Verification items for the finished model (mm, model axes). Face numbers are marked on the shaded views. Give positions to 0.01 mm unless a question says otherwise; leave off trailing zeros. Write each loop counter-clockwise with the first axis right and the second up, starting at its lowest first coordinate (ties: lowest second). Pieces come first, ordered by that corner, then holes. Notation, with made-up numbers: (41, -0.5) -> (53, -0.5) arc R21 cw to (53, 16.5) -> close; hole circle Ø6 at (-13, 8). An arc over 180 degrees is marked (long way). Use one line per item in the form item = value. Start each with the question number.
(1) Depth check by flat-ended pin: pin 1 Ø3 at (x, y) = (403.5, 101) entering from +Z. Enter the tip coordinate at first touch or a pass-through.
(2) Scan lines: L1, parallel to Y at x = 25, z = 4.9; L2, parallel to Y at x = 25, z = 2.05; L3, parallel to Y at x = 335, z = 0.75. Record each from-to range of solid material in increasing order.
(3) Section check A-A, the plane y = 50. Record the cut outline in (x, z).
(4) Release check for a two-part mould opening along Z. For the marked faces 1 and 2 record: pulls with the +Z half, pulls with the -Z half, needs draft (parallel to the pull), parting line crosses it, or undercut.
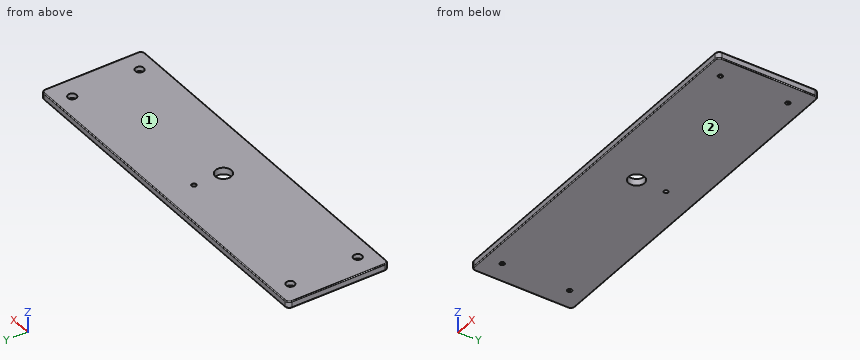
from build123d import *

# Parameters (mm, degrees)
SKETCH1_W                                           = 430
SKETCH1_H                                           = 120
EXTRUDE1_DEPTH                                      = 8
FILLET1_R                                           = 5
FILLET2_R                                           = 1
F_5_0_5_DIAMETER_HOLE1_D                            = 5
F_19_0_19_DIAMETER_HOLE1_D                          = 19
CHAMFER1_SIZE                                       = 0.25
CHAMFER1_SIZE2                                      = 0.144337567
CBORE_FOR_M5_HEX_SOCKET_HEAD_CAP_SCREW1_D           = 5.5
CBORE_FOR_M5_HEX_SOCKET_HEAD_CAP_SCREW1_CBORE_D     = 10
CBORE_FOR_M5_HEX_SOCKET_HEAD_CAP_SCREW1_CBORE_DEPTH = 5.4


with BuildPart() as part:
    # Sketch1 → Extrude1 (new body)
    with BuildSketch(Plane.XY):
        with Locations((215, 60)):
            Rectangle(SKETCH1_W, SKETCH1_H)
    extrude(amount=EXTRUDE1_DEPTH)

    # Fillet1
    fillet1_edges = [part.edges().sort_by_distance(p)[0] for p in [
        (0, 120, 4),
        (430, 120, 4),
        (430, 0, 4),
        (0, 0, 4),
    ]]
    fillet(fillet1_edges, radius=FILLET1_R)

    # Fillet2
    fillet2_edges = [part.edges().sort_by_distance(p)[0] for p in [
        (215, 0, 0),
        (215, 0, 8),
        (0, 60, 0),
        (215, 120, 0),
        (430, 60, 0),
        (1.464466094, 118.535533906, 0),
        (428.535533906, 118.535533906, 0),
        (428.535533906, 1.464466094, 0),
        (1.464466094, 1.464466094, 0),
        (0, 60, 8),
        (430, 60, 8),
        (215, 120, 8),
        (1.464466094, 118.535533906, 8),
        (428.535533906, 118.535533906, 8),
        (428.535533906, 1.464466094, 8),
        (1.464466094, 1.464466094, 8),
    ]]
    fillet(fillet2_edges, radius=FILLET2_R)

    # Ø5.0 (5) Diameter Hole1 (through all)
    with Locations(Plane(origin=(215, 85, 8), x_dir=(1, 0, 0), z_dir=(0, 0, 1))):
        with Locations((0, 0)):
            Hole(F_5_0_5_DIAMETER_HOLE1_D / 2)

    # Ø19.0 (19) Diameter Hole1 (through all)
    with Locations(Plane(origin=(215, 50, 8), x_dir=(1, 0, 0), z_dir=(0, 0, 1))):
        with Locations((0, 0)):
            Hole(F_19_0_19_DIAMETER_HOLE1_D / 2)

    # Chamfer1
    chamfer1_edges = [part.edges().sort_by_distance(p)[0] for p in [
        (217.5, 85, 8),
    ]]
    chamfer1_side = [part.faces().sort_by_distance(p)[0] for p in [
        (215, 60.046713467, 8),
    ]]
    chamfer(chamfer1_edges, length=CHAMFER1_SIZE, length2=CHAMFER1_SIZE2, reference=chamfer1_side[0])

    # CBORE for M5 Hex Socket Head Cap Screw1 (through all)
    with Locations(Plane(origin=(25, 20, 8), x_dir=(1, 0, 0), z_dir=(0, 0, 1))):
        with Locations((0, 0), (0, 80), (380, 0), (380, 80)):
            CounterBoreHole(CBORE_FOR_M5_HEX_SOCKET_HEAD_CAP_SCREW1_D / 2, CBORE_FOR_M5_HEX_SOCKET_HEAD_CAP_SCREW1_CBORE_D / 2, CBORE_FOR_M5_HEX_SOCKET_HEAD_CAP_SCREW1_CBORE_DEPTH)


solid = part.part
Completed:
q1.pin_1 = 2.6
q2.L1 = 0 to 15, 25 to 95, 105 to 120
q2.L2 = 0 to 17.25, 22.75 to 97.25, 102.75 to 120
q2.L3 = 0.03 to 119.97
q3.outline = (0, 1) arc R1 ccw to (1, 0) -> (205.5, 0) -> (205.5, 8) -> (1, 8) arc R1 ccw to (0, 7) -> close; (224.5, 0) -> (429, 0) arc R1 ccw to (430, 1) -> (430, 7) arc R1 ccw to (429, 8) -> (224.5, 8) -> close
q4.face_1 = pulls with the +Z half
q4.face_2 = pulls with the -Z half
